Could you check a few things on this model? Use its own coordinates, in mm. A direction names the side the tool comes from. Round coordinates to 2 decimals unless told otherwise and drop trailing zeros. Order: outer loops, then holes, each group sorted by start corner. A loop starts at its lowest first (then second) coordinate and runs counter-clockwise, first axis right, second up.
```python
from build123d import *

# Parameters (mm, degrees)
SKETCH1_R           = 10.6934
BOSS_EXTRUDE1_DEPTH = 50.8
FILLET1_R           = 7.62
SKETCH2_R           = 1.95
CUT_EXTRUDE1_DEPTH  = 90.044185298
CUT_EXTRUDE3_REACH  = 82.692
SKETCH3_R           = 1.5


with BuildPart() as part:
    # Sketch1 → Boss-Extrude1 (new body)
    with BuildSketch(Plane(origin=(0, 0, 0), x_dir=(1, 0, 0), z_dir=(0, 1, 0))):
        with BuildLine():
            Line((-27.575797838, -21.068578528), (-27.575797838, -27.418578528))
            Line((-27.575797838, -27.418578528), (-17.415797838, -27.418578528))
            ThreePointArc((-17.415797838, -27.418578528), (14.781852954, -31.694178295), (7.137192233, -0.126336551))
            Line((7.137192233, -0.126336551), (7.137192233, 20.467104736))
            ThreePointArc((7.137192233, 20.467104736), (0.787192233, 46.664739041), (-5.562807767, 20.467104736))
            Line((-5.562807767, 20.467104736), (-5.562807767, 0.310008465))
            ThreePointArc((-5.562807767, 0.310008465), (-12.507890511, -3.450714702), (-17.415797838, -9.638578528))
            Line((-17.415797838, -9.638578528), (-27.575797838, -9.638578528))
            Line((-27.575797838, -9.638578528), (-27.575797838, -15.988578528))
            Line((-27.575797838, -15.988578528), (-16.166011022, -15.988578528))
            ThreePointArc((-16.166011022, -15.988578528), (16.657434353, -18.528578528), (-16.166011022, -21.068578528))
            Line((-16.166011022, -21.068578528), (-27.575797838, -21.068578528))
        make_face()
        with Locations(Location((0.787192233, 32.796339041, 0), (0, 0, 270))):
            Circle(SKETCH1_R, mode=Mode.SUBTRACT)
    extrude(amount=BOSS_EXTRUDE1_DEPTH)

    # Fillet1
    fillet1_edges = [part.edges().sort_by_distance(p)[0] for p in [
        (-5.562807767, 25.4, -0.310008465),
        (7.137192233, 25.4, 0.126336551),
        (-5.562807767, 25.4, -20.467104736),
        (7.137192233, 25.4, -20.467104736),
    ]]
    fillet(fillet1_edges, radius=FILLET1_R)

    # Sketch2 → Cut-Extrude1 (cut, through all)
    with BuildSketch(Plane(origin=(0, 0, 21.068578528), x_dir=(-1, 0, 0), z_dir=(0, 0, -1))):
        with Locations((22.495797838, 40.64)):
            Circle(SKETCH2_R)
        with Locations(Location((22.495797838, 10.16, 0), (0, 0, 180))):
            Circle(SKETCH2_R)
    extrude(amount=-CUT_EXTRUDE1_DEPTH, mode=Mode.SUBTRACT)

    # Sketch3 → Cut-Extrude3 (cut, up to next)
    with BuildSketch(Plane(origin=(0, 0, 9.638578528), x_dir=(-1, 0, 0), z_dir=(0, 0, -1)), mode=Mode.PRIVATE) as cut_extrude3_sk1:
        with Locations((22.495797838, 10.16)):
            Circle(SKETCH3_R)
    cut_extrude3_tool1 = extrude(cut_extrude3_sk1.sketch, amount=-CUT_EXTRUDE3_REACH, mode=Mode.PRIVATE) & part.part
    # Sketch3 → Cut-Extrude3 (cut, up to next)
    with BuildSketch(Plane(origin=(0, 0, 9.638578528), x_dir=(-1, 0, 0), z_dir=(0, 0, -1)), mode=Mode.PRIVATE) as cut_extrude3_sk2:
        with Locations((22.495797838, 40.64)):
            Circle(SKETCH3_R)
    cut_extrude3_tool2 = extrude(cut_extrude3_sk2.sketch, amount=-CUT_EXTRUDE3_REACH, mode=Mode.PRIVATE) & part.part
    add(cut_extrude3_tool1.solids().sort_by_distance((-22.495798, 10.16, 9.638579))[0], mode=Mode.SUBTRACT)
    add(cut_extrude3_tool2.solids().sort_by_distance((-22.495798, 40.64, 9.638579))[0], mode=Mode.SUBTRACT)


solid = part.part
```
Q1. For faces 5 (the cylindrical face through (-14, 25.04, 4.84)), 6 (the cylindrical face through (-23.93, 8.84, 24.2)), 7 (the cylindrical face through (8.107, 25.756, -0.818)), 8 (the flat face through (-2, 50.8, -4)), 9 (the cylindrical face through (16.643, 25.044, 17.838)), which set-ups out of +Z, -Z, +X, -X, +Y, -Y let a thin tool reach every point of the face, with its end or its side?
Q2. Imagine slicing it at A-A, the plane z = 14. Please give me the cut outline in (x, y).
Q3. I need wall thicknesses on L1, parallel to X at y = 40, z = 12; L2, parallel to Z at x = -7, y = 26; L3, parallel to Z at x = -21.5, y = 13. Which ranges of each line are inside material? Lowest first, please.
Q4. Imagine slicing it at C-C, the plane x = -4. Please give me the cut outline in (y, z).
Q5. Imagine slicing it at B-B, the plane y = 40.64. Please give me the cut outline in (x, z) (3 decimals).
Q6. Imagine slicing it at D-D, the plane z = 25. Please give me the cut outline in (x, y).
Q7. For P1, Ø3, axis at x = -24.5, y = 16.5, coming from the +Z side; P2, Ø5.5, axis at y = 31, z = -10.5, coming from the -X side; P3, Ø4, axis at x = -21, y = 21, coming from the -Z side; P4, Ø1.8, axis at x = -22.5, y = 10.16, coming from the +Z side, each with a flat end and sliding along its axis, tell me the tip position at first contact or that it passes through.
Q8. We'd pull the mould along X, two halves only. Please class faces 1 (the cylindrical face through (-21.305, 39.727, 12.769)), 2 (the flat face through (-23, 25, 27.419)), 3 (the flat face through (-27.576, 25, 13)), 4 (the cylindrical face through (1.26, 25.044, -46.657)): released by +X, released by -X, zero draft, split by the parting line, or undercut.
Filled in:
1. face 5: -X, +Y, -Y
1. face 6: +Z
1. face 7: +X, +Y, -Y
1. face 8: +Z, -Z, +X, -X, +Y
1. face 9: +Y, -Y
2. outline: (-27.58, 0) - (-15.73, 0) - (-15.73, 50.8) - (-27.58, 50.8) - close; (16.02, 0) - (19.3, 0) - (19.3, 50.8) - (16.02, 50.8) - close; hole circle Ø3 at (-22.5, 10.16); hole circle Ø3 at (-22.5, 40.64)
3. L1: x = -27.58 to -23.85, -21.14 to -15.02, 15.31 to 18.72
3. L2: z = -44.27 to -40.12, -25.47 to -20.92, -0.85 to 3.65, 33.41 to 36.87
3. L3: z = 9.64 to 15.99, 21.07 to 27.42
4. outline: (0, -45.81) - (50.8, -45.81) - (50.8, -42.36) - (0, -42.36) - close; (0, -23.23) - (50.8, -23.23) - (50.8, 2.55) - (0, 2.55) - close; (0, 34.51) - (50.8, 34.51) - (50.8, 37.77) - (0, 37.77) - close
5. outline: (-27.576, 9.639) - (-23.996, 9.639) - (-23.996, 15.989) - (-27.576, 15.989) - close; (-27.576, 21.069) - (-24.446, 21.069) - (-24.446, 27.419) - (-27.576, 27.419) - close; (-20.996, 9.639) - (-17.416, 9.639) arc R19.685 ccw to (-9.463, 1.349) arc R7.62 cw to (-5.563, -5.301) - (-5.563, -16.469) arc R7.62 cw to (-8.229, -22.259) arc R13.868 ccw (long way) to (9.803, -22.259) arc R7.62 cw to (7.137, -16.469) - (7.137, -4.539) arc R7.62 cw to (10.68, 1.898) arc R19.685 ccw (long way) to (-17.416, 27.419) - (-20.546, 27.419) - (-20.546, 21.069) - (-16.166, 21.069) arc R16.51 cw (long way) to (-16.166, 15.989) - (-20.996, 15.989) - close; hole circle Ø21.387 at (0.787, -32.796)
6. outline: (-27.58, 0) - (-15.04, 0) - (-15.04, 50.8) - (-27.58, 50.8) - close; (15.34, 0) - (18.74, 0) - (18.74, 50.8) - (15.34, 50.8) - close; hole circle Ø3.9 at (-22.5, 10.16); hole circle Ø3.9 at (-22.5, 40.64)
7. P1: stops at z = 27.42
7. P2: stops at x = -5.56
7. P3: stops at z = 9.64
7. P4: passes through
8. face 1: undercut
8. face 2: zero draft
8. face 3: released by -X
8. face 4: split by the parting line
